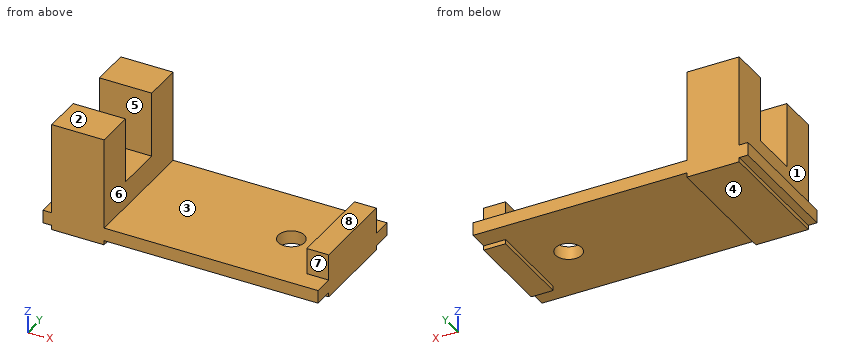
from build123d import *

# Parameters (mm, degrees)
F0_W     = 6
F0_H     = 4.5
F0_H_2   = 5.5
F0_R     = 1.5
F0_W_2   = 2.5
F0_H_3   = 10
F1_DEPTH = 1.5
F2_DEPTH = 3
F3_DEPTH = 10.5
F4_DEPTH = 2


with BuildPart() as f1:
    # F0 (on Top) → F1 (new body)
    with BuildSketch(Plane.XY):
        Polygon((0, 14.5), (0, 0), (1, 0), (1, 4.5), (1, 10), (1, 14.5), align=None)
        with Locations((4, 12.25)):
            Rectangle(F0_W, F0_H)
        with Locations((4, 7.25)):
            Rectangle(F0_W, F0_H_2)
        with Locations((4, 2.25)):
            Rectangle(F0_W, F0_H)
        Polygon((7, 4.5), (7, 0), (31.5, 0), (31.5, 2.25), (29, 2.25), (29, 12.25), (31.5, 12.25), (31.5, 14.5), (7, 14.5), (7, 10), align=None)
        with Locations((24.5, 7.25)):
            Circle(F0_R, mode=Mode.SUBTRACT)
        with Locations((30.25, 7.25)):
            Rectangle(F0_W_2, F0_H_3)
    extrude(amount=-F1_DEPTH)

    # F0 (on Top) → F2 (join)
    with BuildSketch(Plane.XY):
        with Locations((30.25, 7.25)):
            Rectangle(F0_W_2, F0_H_3)
        with Locations((4, 12.25)):
            Rectangle(F0_W, F0_H)
        with Locations((4, 7.25)):
            Rectangle(F0_W, F0_H_2)
        with Locations((4, 2.25)):
            Rectangle(F0_W, F0_H)
    extrude(amount=F2_DEPTH)

    # F0 (on Top) → F3 (join)
    with BuildSketch(Plane.XY):
        with Locations((4, 12.25)):
            Rectangle(F0_W, F0_H)
        with Locations((4, 2.25)):
            Rectangle(F0_W, F0_H)
    extrude(amount=F3_DEPTH)

    # F0 (on Top) → F4 (join)
    with BuildSketch(Plane.XY):
        with Locations((4, 12.25)):
            Rectangle(F0_W, F0_H)
        with Locations((4, 7.25)):
            Rectangle(F0_W, F0_H_2)
        with Locations((4, 2.25)):
            Rectangle(F0_W, F0_H)
        with Locations((30.25, 7.25)):
            Rectangle(F0_W_2, F0_H_3)
    extrude(amount=-F4_DEPTH)


solid = f1.part
Design review of the part built by this model. Coordinates are the model's own, in mm. Face numbers are marked on the shaded views. A direction names the side the tool comes from. Coordinates: 2 decimals unless noted, no trailing zeros. Order: outer loops, then holes, each group sorted by start corner. A loop starts at its lowest first (then second) coordinate and runs counter-clockwise, first axis right, second up. Notation, with made-up numbers: (64.25, -25) -> (68.25, -25) arc R22 cw to (68.25, 0) -> close; hole circle Ø1 at (-4, 40). An arc over 180 degrees is marked (long way). Use one line per item in the form item = value. Start each with the question number.
(1) Add section C-C on x = 24.5. State the section outline as (y, z) points.
(2) For probe 1 along X at (y, z) = (12, 2); probe 2 along Y at (x, z) = (24.5, -0.55); probe 3 along Y at (x, z) = (5.5, 7.75), list the stretches that pass through material, from the lowest coordinate up.
(3) The part is to be moulded in two halves that separate along X. For the marked faces 1, 2 and 3, say which applies: +X half, -X half, draft (parallel to the pull), parting line (faces both ways), or undercut.
(4) For the marked faces 4, 5, 6, 7 and 8, list the 3-axis set-ups (+Z, -Z, +X, -X, +Y, -Y) from which the entire face can be reached by the end or side of a thin tool; tool diameter is ignored.
(5) Add section A-A on z = 2.5. State the section outline as (x, y) points.
(6) Insertion check: pin 1 (0.8 mm diameter, centred on x = 31, z = 2, fed in from +Y); pin 2 (1.2 mm diameter, centred on x = 30.5, y = 5.5, fed in from +Z); pin 3 (0.5 mm diameter, centred on x = 0.5, y = 10.5, fed in from +Z). Each pin has a flat end and moves straight along its axis. Give the tip position at first contact, or say it passes through.
(7) Add section D-D on x = 4. State the section outline as (y, z) points.
(8) Add section B-B on y = 7.25. State the section outline as (x, z) points.
Answer block:
q1.outline = (0, -1.5) -> (5.75, -1.5) -> (5.75, 0) -> (0, 0) -> close; (8.75, -1.5) -> (14.5, -1.5) -> (14.5, 0) -> (8.75, 0) -> close
q2.probe_1 = 1 to 7, 29 to 31.5
q2.probe_2 = 0 to 5.75, 8.75 to 14.5
q2.probe_3 = 0 to 4.5, 10 to 14.5
q3.face_1 = -X half
q3.face_2 = draft
q3.face_3 = undercut
q4.face_4 = -Z, +X, -X, +Y, -Y
q4.face_5 = +Z, +X, -X
q4.face_6 = +Z, +Y, -Y
q4.face_7 = +Z, +X, -Y
q4.face_8 = +Z, +X, +Y, -Y
q5.outline = (1, 0) -> (7, 0) -> (7, 14.5) -> (1, 14.5) -> close; (29, 2.25) -> (31.5, 2.25) -> (31.5, 12.25) -> (29, 12.25) -> close
q6.pin_1 = 12.25
q6.pin_2 = 3
q6.pin_3 = 0
q7.outline = (0, -2) -> (14.5, -2) -> (14.5, 10.5) -> (10, 10.5) -> (10, 3) -> (4.5, 3) -> (4.5, 10.5) -> (0, 10.5) -> close
q8.outline = (0, -1.5) -> (1, -1.5) -> (1, -2) -> (7, -2) -> (7, -1.5) -> (23, -1.5) -> (23, 0) -> (7, 0) -> (7, 3) -> (1, 3) -> (1, 0) -> (0, 0) -> close; (26, -1.5) -> (29, -1.5) -> (29, -2) -> (31.5, -2) -> (31.5, 3) -> (29, 3) -> (29, 0) -> (26, 0) -> close
